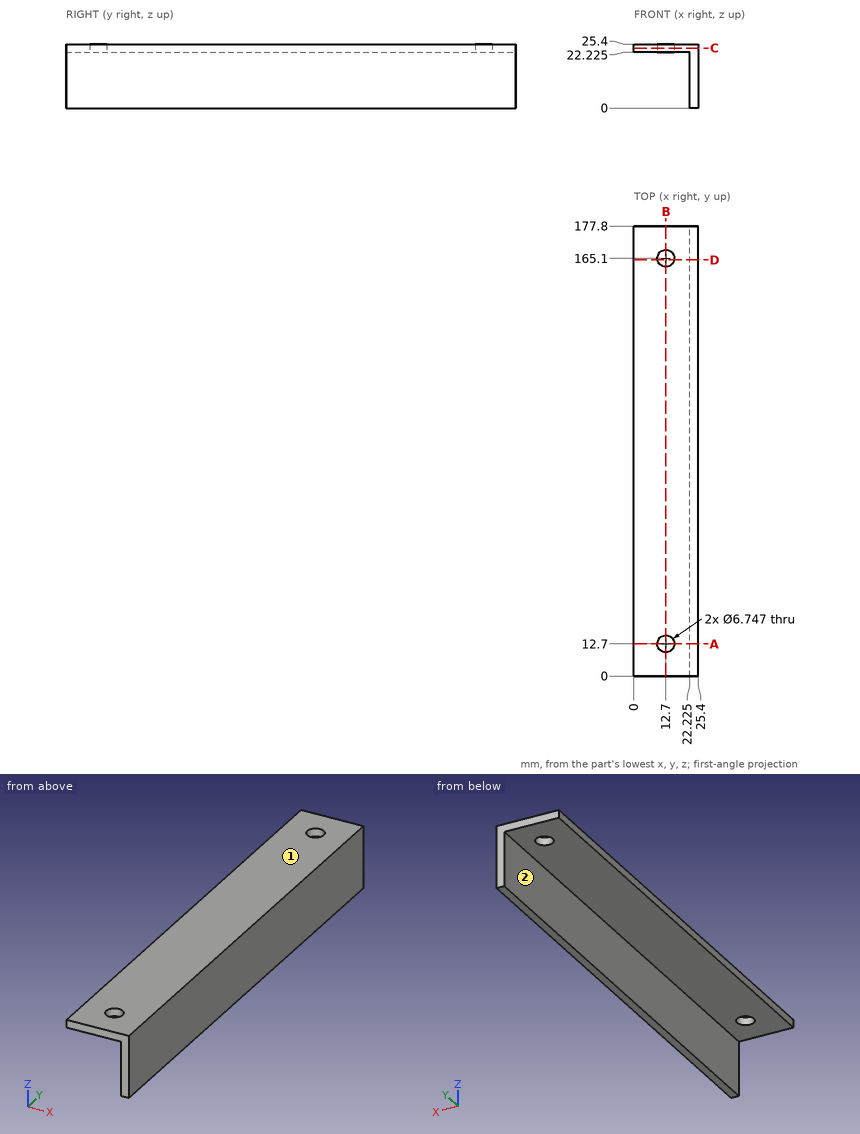
Source: three-view drawing plus pictorial views. Frame: mm from the lowest corner of the part. A direction names the side the tool comes from. Coordinates: 2 decimals unless noted, no trailing zeros. Write each loop counter-clockwise with the first axis right and the second up, starting at its lowest first coordinate (ties: lowest second). Pieces come first, ordered by that corner, then holes. Notation, with made-up numbers: (48, -13) - (96, -13) arc R14 ccw to (96, 2) - close; hole circle Ø1 at (82, 51.5). An arc over 180 degrees is marked (long way). Answer as a JSON object with one key per item and string values.
Q1. Section query D-D, the plane y = 164.5. Output: boundary loops of the cut face in (x, z) (1 decimal), plus the area to 3 significant figures.
Ans:
{"outline": "(0, 22.2) - (9.4, 22.2) - (9.4, 25.4) - (0, 25.4) - close; (16, 22.2) - (22.2, 22.2) - (22.2, 0) - (25.4, 0) - (25.4, 25.4) - (16, 25.4) - close", "area": "130 mm2"}
Q2. Material intervals for line 1 (Y direction, x = 12.7, z = 23.65); line 2 (X direction, y = 12.7, z = 24.55); line 3 (X direction, y = 78.5, z = 16.5) (3 decimals), sorted ascending. Write a range as [from, to].
Ans:
{"line 1": "y = [0, 9.33], [16.07, 161.73], [168.47, 177.8]", "line 2": "x = [0, 9.33], [16.07, 25.4]", "line 3": "x = [22.225, 25.4]"}
Q3. Section query C-C, the plane z = 23.75. Output: boundary loops of the cut face in (x, y).
Ans:
{"outline": "(0, 0) - (25.4, 0) - (25.4, 177.8) - (0, 177.8) - close; hole circle Ø6.75 at (12.7, 12.7); hole circle Ø6.75 at (12.7, 165.1)"}
Q4. Set-up query: the marked faces 1 and 2. Return all of +Z, -Z, +X, -X, +Y, -Y with unobstructed straight access to the full face (end or side cutting, diameter ignored); none if empty.
Ans:
{"face 1": "+Z, +X, -X, +Y, -Y", "face 2": "-Z, -X, +Y, -Y"}
Q5. First-contact query: pin 1 Ø10 at (x, y) = (9.5, 90.5) entering from -Z (3 decimals); pin 2 Ø5.5 at (x, y) = (12.7, 12.7) entering from -Z. Flat tips, straight axial feed; report the tip coordinate or a pass-through.
Ans:
{"pin 1": "stops at z = 22.225", "pin 2": "passes through"}
Q6. Section query B-B, the plane x = 12.7. Output: boundary loops of the cut face in (y, z) (1 decimal).
Ans:
{"outline": "(0, 22.2) - (9.3, 22.2) - (9.3, 25.4) - (0, 25.4) - close; (16.1, 22.2) - (161.7, 22.2) - (161.7, 25.4) - (16.1, 25.4) - close; (168.5, 22.2) - (177.8, 22.2) - (177.8, 25.4) - (168.5, 25.4) - close"}
Q7. Section query A-A, the plane y = 12.7. Output: boundary loops of the cut face in (x, z) (1 decimal).
Ans:
{"outline": "(0, 22.2) - (9.3, 22.2) - (9.3, 25.4) - (0, 25.4) - close; (16.1, 22.2) - (22.2, 22.2) - (22.2, 0) - (25.4, 0) - (25.4, 25.4) - (16.1, 25.4) - close"}
